from build123d import *

# Parameters (mm, degrees)
SKETCH_1_W          = 40
SKETCH_1_H          = 69
EXTRUDE_1_DEPTH     = 20
SKETCH_2_R          = 8
CUT_EXTRUDE_1_DEPTH = 20
SKETCH_3_W          = 40
SKETCH_3_H          = 20
EXTRUDE_2_DEPTH     = 26
SKETCH_8_W          = 15.4
SKETCH_8_H          = 15.4
CUT_EXTRUDE_6_DEPTH = 100
SKETCH_4_R          = 1.65
CUT_EXTRUDE_2_DEPTH = 40
SKETCH_5_W          = 5
SKETCH_5_H          = 5
CUT_EXTRUDE_3_DEPTH = 6
FILLET_1_R          = 2
SKETCH_6_W          = 16
SKETCH_6_H          = 24
CUT_EXTRUDE_4_DEPTH = 50
SKETCH_7_R          = 4
CUT_EXTRUDE_5_DEPTH = 100
FILLET_2_R          = 1
SKETCH_9_R          = 1.65
CUT_EXTRUDE_7_DEPTH = 1000


with BuildPart() as part:
    # 草图1 → 凸台-拉伸1 (new body)
    with BuildSketch(Plane.XY):
        Rectangle(SKETCH_1_W, SKETCH_1_H)
    extrude(amount=EXTRUDE_1_DEPTH)

    # 草图2 → 切除-拉伸1 (cut)
    with BuildSketch(Plane.XY.offset(20)):
        Circle(SKETCH_2_R)
    extrude(amount=-CUT_EXTRUDE_1_DEPTH, mode=Mode.SUBTRACT)

    # 草图3 → 凸台-拉伸2 (add)
    with BuildSketch(Plane.XZ.offset(34.5)):
        with Locations((0, 10)):
            Rectangle(SKETCH_3_W, SKETCH_3_H)
    extrude(amount=EXTRUDE_2_DEPTH)

    # 草图8 → 切除-拉伸6 (cut)
    with BuildSketch(Plane.XY.offset(20)):
        with Locations((0, -31.5)):
            Rectangle(SKETCH_8_W, SKETCH_8_H)
    extrude(amount=-CUT_EXTRUDE_6_DEPTH, mode=Mode.SUBTRACT)

    # 草图4 → 切除-拉伸2 (cut)
    with BuildSketch(Plane.XY.offset(20)):
        with Locations((4.5, -49.2)):
            Circle(SKETCH_4_R)
        with Locations((-4.5, -49.2)):
            Circle(SKETCH_4_R)
    extrude(amount=-CUT_EXTRUDE_2_DEPTH, mode=Mode.SUBTRACT)

    # 草图5 → 切除-拉伸3 (cut)
    with BuildSketch(Plane.XZ.offset(60.5)):
        with Locations((0, 12)):
            Rectangle(SKETCH_5_W, SKETCH_5_H)
    extrude(amount=-CUT_EXTRUDE_3_DEPTH, mode=Mode.SUBTRACT)

    # 圆角1
    fillet_1_edges = [part.edges().sort_by_distance(p)[0] for p in [
        (-20, 34.5, 10),
        (20, 34.5, 10),
    ]]
    fillet(fillet_1_edges, radius=FILLET_1_R)

    # 草图6 → 切除-拉伸4 (cut)
    with BuildSketch(Plane.XY.offset(20)):
        with Locations((0, 22.5)):
            Rectangle(SKETCH_6_W, SKETCH_6_H)
    extrude(amount=-CUT_EXTRUDE_4_DEPTH, mode=Mode.SUBTRACT)

    # 草图7 → 切除-拉伸5 (cut)
    with BuildSketch(Plane(origin=(20, 0, 0), x_dir=(0, 0, -1), z_dir=(1, 0, 0))):
        with Locations((-10, 24.5)):
            Circle(SKETCH_7_R)
    extrude(amount=-CUT_EXTRUDE_5_DEPTH, mode=Mode.SUBTRACT)

    # 圆角2
    fillet_2_edges = [part.edges().sort_by_distance(p)[0] for p in [
        (-8, 34.5, 10),
        (8, 34.5, 10),
        (8, 10.5, 10),
        (-8, 10.5, 10),
    ]]
    fillet(fillet_2_edges, radius=FILLET_2_R)

    # 草图9 → 切除-拉伸7 (cut)
    with BuildSketch(Plane(origin=(20, 0, 0), x_dir=(0, 0, -1), z_dir=(1, 0, 0))):
        with Locations((-10, -31.5)):
            Circle(SKETCH_9_R)
    extrude(amount=-CUT_EXTRUDE_7_DEPTH, mode=Mode.SUBTRACT)


solid = part.part
Design review of the part built by this model. Coordinates are the model's own, in mm. A direction names the side the tool comes from. Give positions to 0.01 mm unless a question says otherwise; leave off trailing zeros. Write each loop counter-clockwise with the first axis right and the second up, starting at its lowest first coordinate (ties: lowest second). Pieces come first, ordered by that corner, then holes. Notation, with made-up numbers: M -14,-29.75 L 36,-29.75 A23 cw 36,-0.75 Z; hole C 62.5,-16.5 d11. An arc over 180 degrees is marked long. Answer as a JSON object with one key per item and string values. Group by question number.
1) Clearance check with flat-ended pins moving along their axes: pin 1 Ø2 at (y, z) = (-32, 10) entering from -X; pin 2 Ø2.5 at (x, z) = (0, 12.5) entering from -Y; pin 3 Ø7 at (x, z) = (1, 9) entering from +Y. State where each tip first meets the part, or that it passes through.
2) For line 1 along Y through (x, z) = (-13.75, 10); line 2 along X through (y, z) = (-32, 14.5); line 3 along Y through (x, z) = (-17, 8.5), list the stretches that pass through material, from the lowest coordinate up.
3) Mouldability with a two-part tool opening along Z and no side actions: class faces 4 (the face through (-19.43, 33.9, 10.14)), 5 (the face through (-13.916, 28.466, 10.521)), 6 (the face through (0, -12, 20)), 7 (the face through (0, -12, 0)) as released by +Z, released by -Z, zero draft, split by the parting line, or undercut.
4) Tool access review of faces 1 (the face through (7.7, -33.3, 10.1)), 2 (the face through (8, 20, 10)), 3 (the face through (0, -54.5, 12)): name each direction out of +Z, -Z, +X, -X, +Y, -Y from which nothing blocks a thin tool from reaching the whole face with its end or side.
5) We need section B-B (y = -49.2). Give the boundary of the cut face in (x, z), and give its area (3 significant figures).
6) We need section C-C (z = 3.5). Give the boundary of the cut face in (x, y), and give its area (3 significant figures).
7) We need section A-A (y = -27). Give the boundary of the cut face in (x, z), and give its area (3 significant figures).
8) We need section D-D (x = 4.5). Give the boundary of the cut face in (y, z).
Answer key:
{
 "1": {"pin 1": "passes through", "pin 2": "stops at y = -54.5", "pin 3": "stops at y = 10.5"},
 "2": {"line 1": "y = -60.5 to -33.15, -29.85 to 20.5, 28.5 to 34.5", "line 2": "x = -20 to -7.7, 7.7 to 20", "line 3": "y = -60.5 to -32.19, -30.81 to 20.79, 28.21 to 34.5"},
 "3": {"face 4": "zero draft", "face 5": "undercut", "face 6": "released by +Z", "face 7": "released by -Z"},
 "4": {"face 1": "+Z, -Z", "face 2": "+Z, -Z, +Y", "face 3": "-Y"},
 "5": {"outline": "M -20,0 L -6.15,0 L -6.15,20 L -20,20 Z; M -2.85,0 L 2.85,0 L 2.85,20 L -2.85,20 Z; M 6.15,0 L 20,0 L 20,20 L 6.15,20 Z", "area": "668 mm²"},
 "6": {"outline": "M -20,-60.5 L 20,-60.5 L 20,32.5 A2 ccw 18,34.5 L 9,34.5 A1 ccw 8,33.5 L 8,11.5 A1 cw 7,10.5 L -7,10.5 A1 cw -8,11.5 L -8,33.5 A1 ccw -9,34.5 L -18,34.5 A2 ccw -20,32.5 Z; hole C 0,0 d16; hole M -7.7,-39.2 L 7.7,-39.2 L 7.7,-23.8 L -7.7,-23.8 Z; hole C -4.5,-49.2 d3.3; hole C 4.5,-49.2 d3.3", "area": "2,960 mm²"},
 "7": {"outline": "M -20,0 L -7.7,0 L -7.7,20 L -20,20 Z; M 7.7,0 L 20,0 L 20,20 L 7.7,20 Z", "area": "492 mm²"},
 "8": {"outline": "M -60.5,0 L -50.85,0 L -50.85,20 L -60.5,20 Z; M -47.55,0 L -39.2,0 L -39.2,20 L -47.55,20 Z; M -23.8,0 L -6.61,0 L -6.61,20 L -23.8,20 Z; M 6.61,0 L 10.5,0 L 10.5,20 L 6.61,20 Z"}
}
